Part print with two shaded views. Sizes in mm from the minimum x, y, z corner. Give positions to 0.01 mm unless a question says otherwise; leave off trailing zeros. Order: outer loops, then holes, each group sorted by start corner. A loop starts at its lowest first (then second) coordinate and runs counter-clockwise, first axis right, second up. Notation, with made-up numbers: (29.5, -9.75) -> (50.5, -9.75) arc R26 cw to (50.5, 9.25) -> close; hole circle Ø6 at (62.5, 46). An arc over 180 degrees is marked (long way). Answer in a Markdown table with one row per item. Add a question column.
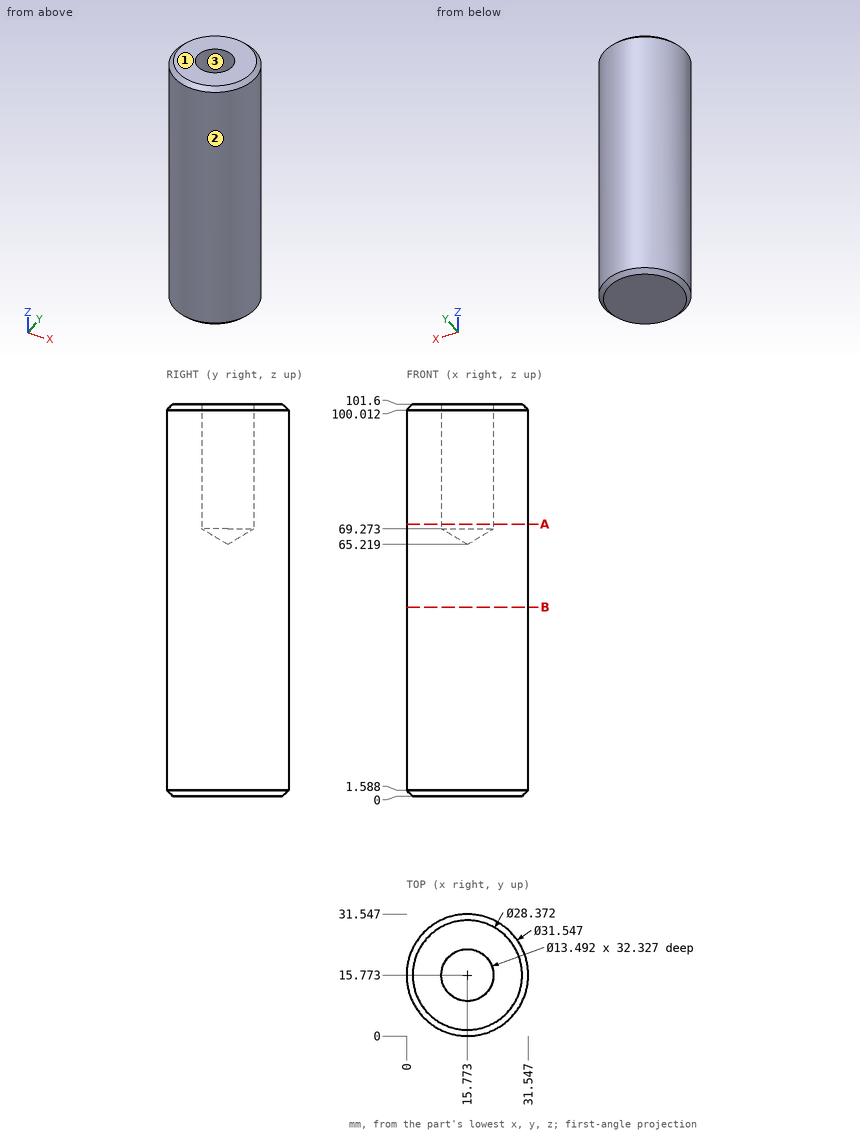
Item 1: Wall check: line 1 (X direction, y = 20, z = 93.5) (1 decimal); line 2 (Y direction, x = 16, z = 67) (1 decimal); line 3 (X direction, y = 7, z = 83) (1 decimal). Give the ranges that are in metal, low to high.
Item 2: Two-plate mould, pull along X, no slides. Class the marked faces 1, 2 and 3: pulls with the +X half, pulls with the -X half, needs draft (parallel to the pull), parting line crosses it, or undercut.
Item 3: Pin check, flat tips, straight feed: pin 1 Ø12 at (x, y) = (15.77, 15.77) entering from +Z; pin 2 Ø1.5 at (x, z) = (8.5, 33.5) entering from +Y (1 decimal); pin 3 Ø3 at (y, z) = (5, 30) entering from +X. Stop position of each tip, or through.
Item 4: Saw through at B-B on z = 49. List the corners of the cut face in (x, y), plus the area to 3 significant figures.
Item 5: Saw through at A-A on z = 70.5. List the corners of the cut face in (x, y), plus the area to 3 significant figures.
Evaluation:
| question | item | result |
|---|---|---|
| 1 | line 1 | x = 0.6 to 10.5, 21 to 31 |
| 1 | line 2 | y = 0 to 12.8, 18.7 to 31.5 |
| 1 | line 3 | x = 2.7 to 28.9 |
| 2 | face 1 | needs draft |
| 2 | face 2 | parting line crosses it |
| 2 | face 3 | undercut |
| 3 | pin 1 | stops at z = 68.83 |
| 3 | pin 2 | stops at y = 30.1 |
| 3 | pin 3 | stops at x = 28.53 |
| 4 | outline | circle Ø31.55 at (15.77, 15.77) |
| 4 | area | 782 mm2 |
| 5 | outline | circle Ø31.55 at (15.77, 15.77); hole circle Ø13.49 at (15.77, 15.77) |
| 5 | area | 639 mm2 |
